```python
from build123d import *

# Parameters (mm, degrees)
SKETCH_1_R          = 40
EXTRUDE_1_DEPTH     = 300
SKETCH_2_OUTSIDE_W  = 146.124
SKETCH_2_OUTSIDE_H  = 146.124
SKETCH_2_OUTSIDE_R  = 20
CUT_EXTRUDE_1_DEPTH = 150
FILLET_2_R          = 1
FILLET_3_R          = 1
FILLET_4_R          = 1
FILLET_5_R          = 1


with BuildPart() as part:
    # Эскиз1 → Бобышка-Вытянуть1 (new body)
    with BuildSketch(Plane(origin=(0, 0, 0), x_dir=(1, 0, 0), z_dir=(0, 1, 0))):
        with Locations(Location((0, 0, 0), (0, 0, 270))):
            Circle(SKETCH_1_R)
    extrude(amount=EXTRUDE_1_DEPTH)

    # Эскиз2 outside → Вырез-Вытянуть1 (cut)
    with BuildSketch(Plane(origin=(0, 300, 0), x_dir=(1, 0, 0), z_dir=(0, 1, 0))):
        Rectangle(SKETCH_2_OUTSIDE_W, SKETCH_2_OUTSIDE_H)
        with Locations(Location((0, 0, 0), (0, 0, 270))):
            Circle(SKETCH_2_OUTSIDE_R, mode=Mode.SUBTRACT)
    extrude(amount=-CUT_EXTRUDE_1_DEPTH, mode=Mode.SUBTRACT)

    # Скругление2
    fillet_2_edges = [part.edges().sort_by_distance(p)[0] for p in [
        (0, 150, -20),
    ]]
    fillet(fillet_2_edges, radius=FILLET_2_R)

    # Скругление3
    fillet_3_edges = [part.edges().sort_by_distance(p)[0] for p in [
        (0, 300, -20),
    ]]
    fillet(fillet_3_edges, radius=FILLET_3_R)

    # Скругление4
    fillet_4_edges = [part.edges().sort_by_distance(p)[0] for p in [
        (0, 0, -40),
    ]]
    fillet(fillet_4_edges, radius=FILLET_4_R)

    # Скругление5
    fillet_5_edges = [part.edges().sort_by_distance(p)[0] for p in [
        (0, 150, -40),
    ]]
    fillet(fillet_5_edges, radius=FILLET_5_R)


solid = part.part
```
The listing builds one solid part. Answer for the finished solid, in the listing's coordinates (mm). A direction names the side the tool comes from. Coordinates: 2 decimals unless noted, no trailing zeros. Write each loop counter-clockwise with the first axis right and the second up, starting at its lowest first coordinate (ties: lowest second). Pieces come first, ordered by that corner, then holes. Notation, with made-up numbers: (51, -30) - (89, -30) arc R25 cw to (89, 7) - close; hole circle Ø10 at (-29, 52). An arc over 180 degrees is marked (long way). Return JSON: item names as keys, results as strings. Group by question number.
Q1. The part is cut by section A-A on x = 0. Write down the section's boundary in (y, z).
Q2. The part is cut by section D-D on y = 177.5. Write down the section's boundary in (x, z), and give its area (3 significant figures).
Q3. Which of the six approach directions +Z, -Z, +X, -X, +Y, -Y give full straight-line access (tool end or side, diameter ignored) to faces 1 (the flat face through (17, 150, 17)), 2 (the flat face through (1, 0, -1))?
Q4. Find the intervals of material crossed by line 1 along Y through (x, z) = (-6.5, 34.5); line 2 along Z through (x, y) = (0.5, 242); line 3 along X through (y, z) = (257, 11), in increasing order. Write a range as [from, to].
Q5. The part is cut by section B-B on z = 0. Write down the section's boundary in (x, y), and give its area (3 significant figures).
Q6. The part is cut by section C-C on y = 37.5. Write down the section's boundary in (x, z).
Q7. Flat-ended cylindrical pins translate along their axes: pin 1 Ø4 at (x, y) = (-11.5, 174.5) entering from +Z; pin 2 Ø1.5 at (x, z) = (5.5, -23) entering from -Y; pin 3 Ø4 at (x, y) = (19.5, 224.5) entering from -Z; pin 4 Ø6 at (y, z) = (184, 16) entering from -X. Find the tip coordinate at first contact, or state that the pin passes through.
Evaluation:
{
 "1": {"outline": "(0, -39) arc R1 ccw to (1, -40) - (149, -40) arc R1 ccw to (150, -39) - (150, -21) arc R1 cw to (151, -20) - (299, -20) arc R1 ccw to (300, -19) - (300, 19) arc R1 ccw to (299, 20) - (151, 20) arc R1 cw to (150, 21) - (150, 39) arc R1 ccw to (149, 40) - (1, 40) arc R1 ccw to (0, 39) - close"},
 "2": {"outline": "circle Ø40 at (0, 0)", "area": "1,260 mm2"},
 "3": {"face 1": "+Y", "face 2": "+Z, -Z, +X, -X, -Y"},
 "4": {"line 1": "y = [0, 150]", "line 2": "z = [-19.99, 19.99]", "line 3": "x = [-16.7, 16.7]"},
 "5": {"outline": "(-40, 1) arc R1 ccw to (-39, 0) - (39, 0) arc R1 ccw to (40, 1) - (40, 149) arc R1 ccw to (39, 150) - (21, 150) arc R1 cw to (20, 151) - (20, 299) arc R1 ccw to (19, 300) - (-19, 300) arc R1 ccw to (-20, 299) - (-20, 151) arc R1 cw to (-21, 150) - (-39, 150) arc R1 ccw to (-40, 149) - close", "area": "18,000 mm2"},
 "6": {"outline": "circle Ø80 at (0, 0)"},
 "7": {"pin 1": "stops at z = 17.6", "pin 2": "stops at y = 0", "pin 3": "stops at z = -9.68", "pin 4": "stops at x = -15.2"}
}
